The model under review builds one solid part; all positions refer to its coordinate system, in mm. A direction names the side the tool comes from. Coordinates: 2 decimals unless noted, no trailing zeros. Loops run counter-clockwise (first coordinate to the right, second up) from the corner with the lowest first, then second, coordinate; pieces in that order, holes last. Notation, with made-up numbers: M 18,43 L 22,43 A20 cw 22,68 Z; hole C 7.25,-31.75 d10. An arc over 180 degrees is marked long. Write item = value, one per line. Start each with the question number.
Q1. We need section B-B on z = 3.15. Give the boundary of the cut face in (x, y), and give its area (3 significant figures).
Q2. Mouldability with a two-part tool opening along Y and no side actions: class faces 1 (the face through (1.319, 99.985, 2.465)), 2 (the face through (0, -23, 2)), 3 (the face through (26.477, 17.052, 2.465)) as released by +Y, released by -Y, zero draft, split by the parting line, or undercut.
Q3. We need section A-A on y = 63.5. Give the boundary of the cut face in (x, z).
Q4. Clearance check with flat-ended pins moving along their axes: pin 1 Ø2 at (y, z) = (13, 3.5) entering from +X; pin 2 Ø2 at (x, y) = (35.5, 5.5) entering from -Z; pin 3 Ø1 at (y, z) = (74.5, 1.5) entering from -X. State where each tip first meets the part, or that it passes through.
Q5. Wall thickness on probe 1 along Y at (x, z) = (37, 2.1); probe 2 along Y at (x, z) = (-32.5, 1.9); probe 3 along X at (y, z) = (84, 2.95): over which ranges is each line inside the solid? List them lowest first.
Q6. We need section C-C on y = 78.5. Give the boundary of the cut face in (x, z).
Q7. For faces 4 (the face through (26, 53, 5)), 5 (the face through (-32.24, 68.73, 2.46)), list the 3-axis set-ups (+Z, -Z, +X, -X, +Y, -Y) from which the entire face can be reached by the end or side of a thin tool; tool diameter is ignored.
from build123d import *

# Parameters (mm, degrees)
SKETCH2_R           = 10.5
BOSS_EXTRUDE1_DEPTH = 5


with BuildPart() as part:
    # Sketch2 → Boss-Extrude1 (new body)
    with BuildSketch(Plane.XY):
        with BuildLine():
            ThreePointArc((60, 40), (0, 100), (-60, 40))
            ThreePointArc((-60, 40), (-57.988295689, 29.675428199), (-52.2475067, 20.861400806))
            Line((-52.2475067, 20.861400806), (-16.516096513, -16.006828417))
            ThreePointArc((-16.516096513, -16.006828417), (0, -23), (16.516096513, -16.006828417))
            Line((16.516096513, -16.006828417), (52.2475067, 20.861400806))
            ThreePointArc((52.2475067, 20.861400806), (57.988295689, 29.675428199), (60, 40))
        make_face()
        with Locations((32.5, 40)):
            Circle(SKETCH2_R, mode=Mode.SUBTRACT)
        with Locations((-32.5, 40)):
            Circle(SKETCH2_R, mode=Mode.SUBTRACT)
        with BuildLine():
            ThreePointArc((-22.572828784, 83.491003675), (-32.255432897, 68.469423949), (-24.218531469, 52.506689369))
            ThreePointArc((-24.218531469, 52.506689369), (-17.599364702, 41.723678544), (-21.581946383, 29.714276632))
            ThreePointArc((-21.581946383, 29.714276632), (-26.479831206, 17.244012068), (-21.405922791, 4.844325481))
            Line((-21.405922791, 4.844325481), (-8.617093833, -8.351388739))
            ThreePointArc((-8.617093833, -8.351388739), (0, -12), (8.617093833, -8.351388739))
            Line((8.617093833, -8.351388739), (21.405922791, 4.844325481))
            ThreePointArc((21.405922791, 4.844325481), (26.479831206, 17.244012068), (21.581946383, 29.714276632))
            ThreePointArc((21.581946383, 29.714276632), (17.599364702, 41.723678544), (24.218531469, 52.506689369))
            ThreePointArc((24.218531469, 52.506689369), (32.255432897, 68.469423949), (22.572828784, 83.491003675))
            ThreePointArc((22.572828784, 83.491003675), (0, 89), (-22.572828784, 83.491003675))
        make_face(mode=Mode.SUBTRACT)
    extrude(amount=BOSS_EXTRUDE1_DEPTH)


solid = part.part
Returned:
q1.outline = M -60,40 A27.5 ccw -52.25,20.86 L -16.52,-16.01 A23 ccw 16.52,-16.01 L 52.25,20.86 A27.5 ccw 60,40 A60 ccw Z; hole C -32.5,40 d21; hole M -24.22,52.51 A15 cw -21.58,29.71 A18 ccw -21.41,4.84 L -8.62,-8.35 A12 ccw 8.62,-8.35 L 21.41,4.84 A18 ccw 21.58,29.71 A15 cw 24.22,52.51 A18 ccw 22.57,83.49 A49 ccw -22.57,83.49 A18 ccw Z; hole C 32.5,40 d21
q1.area = 5,300 mm^2
q2.face_1 = released by +Y
q2.face_2 = released by -Y
q2.face_3 = undercut
q3.outline = M -55.21,0 L -31.83,0 L -31.83,5 L -55.21,5 Z; M 31.83,0 L 55.21,0 L 55.21,5 L 31.83,5 Z
q4.pin_1 = 45.6
q4.pin_2 = 0
q4.pin_3 = -49.44
q5.probe_1 = 5.13 to 30.51, 49.49 to 87.23
q5.probe_2 = 0.49 to 29.5, 50.5 to 90.44
q5.probe_3 = -40.79 to -21.56, 21.56 to 40.79
q6.outline = M -46.02,0 L -28.54,0 L -28.54,5 L -46.02,5 Z; M 28.54,0 L 46.02,0 L 46.02,5 L 28.54,5 Z
q7.face_4 = +Z, +X, -X, +Y, -Y
q7.face_5 = +Z, -Z
